Source: CAD feature listing. Evaluate the final solid. Frame: model axes, mm. A direction names the side the tool comes from. Coordinates: 2 decimals unless noted, no trailing zeros. Order: outer loops, then holes, each group sorted by start corner. A loop starts at its lowest first (then second) coordinate and runs counter-clockwise, first axis right, second up.
Item 1: Section B-B on y = 52.5. Return the cut outline in (x, z), then the cut area to 3 significant figures.
Item 2: Ray query, line 1 (X direction, y = 29, z = 128); line 2 (Y direction, x = 14.5, z = 134.5); line 3 (Y direction, x = 21, z = 20). Return the intervals inside material, ascending.
Item 3: Contact query for flat-ended pins moving along their axis: P1, Ø4, axis at x = 22.5, z = 61, coming from the -Y side; P2, Ø1, axis at y = 20.5, z = 53, coming from the -X side; P3, Ø10, axis at y = 1, z = 85.5, coming from the +X side; P4, Ø1.5, axis at x = 21.5, z = 58, coming from the +Y side. Output: stop coordinate, or through.
Item 4: Mould query, pull axis X, two halves, no side actions, for faces 1 (the flat face through (20, 25, 81)), 2 (the flat face through (25, 20, 81)), 3 (the flat face through (22, 50, 81)). Classes: released by +X, released by -X, zero draft, split by the parting line, or undercut.
Item 5: Section A-A on x = 14. Return the cut outline in (y, z).
Item 6: Reachability of faces 4 (the flat face through (20, 55, 79)), 5 (the flat face through (20, -10, 79)), 6 (the flat face through (20, 75, 79)), 7 (the flat face through (22, 30, 79)) from +Z, -Z, +X, -X, +Y, -Y: full face, straight path, thin tool, end or side. Return the list, or none.
Item 7: Section C-C on z = 143. Return the cut outline in (x, y).
Item 8: Section D-D on y = 8. Return the cut outline in (x, z).
from build123d import *

# Parameters (mm, degrees)
BOSS_EXTRUDE1_DEPTH      = 160
SKETCH2_W                = 20
SKETCH2_H                = 160
BOSS_EXTRUDE2_DEPTH      = 30
BOSS_EXTRUDE3_DEPTH      = 10
BOSS_EXTRUDE3_DEPTH_BACK = 10
SKETCH3_W                = 5
SKETCH3_H                = 160
BOSS_EXTRUDE4_DEPTH      = 10
BOSS_EXTRUDE4_DEPTH_BACK = 10
SKETCH4_W                = 5
SKETCH4_H                = 160


with BuildPart() as part:
    # Sketch1 → Boss-Extrude1 (new body)
    with BuildSketch(Plane.XY):
        Polygon((0, 0), (20, 0), (20, 20), (10, 20), (10, 60), (20, 60), (20, 80), (0, 80), align=None)
    extrude(amount=BOSS_EXTRUDE1_DEPTH)

    # Sketch2 → Boss-Extrude2 (add)
    with BuildSketch(Plane.XZ):
        with Locations((10, 80)):
            Rectangle(SKETCH2_W, SKETCH2_H)
    extrude(amount=BOSS_EXTRUDE2_DEPTH)

    # Sketch3 → Boss-Extrude3 (add, two sides: drawn at the far end of the back side and taken through both)
    with BuildSketch(Plane(origin=(0, 20, 0), x_dir=(1, 0, 0), z_dir=(0, 1, 0)).offset(-BOSS_EXTRUDE3_DEPTH_BACK)):
        with Locations((22.5, -80)):
            Rectangle(SKETCH3_W, SKETCH3_H)
    extrude(amount=BOSS_EXTRUDE3_DEPTH + BOSS_EXTRUDE3_DEPTH_BACK)

    # Sketch4 → Boss-Extrude4 (add, two sides: drawn at the far end of the back side and taken through both)
    with BuildSketch(Plane.XZ.offset(-60).offset(-BOSS_EXTRUDE4_DEPTH_BACK)):
        with Locations((22.5, 80)):
            Rectangle(SKETCH4_W, SKETCH4_H)
    extrude(amount=BOSS_EXTRUDE4_DEPTH + BOSS_EXTRUDE4_DEPTH_BACK)


solid = part.part
Answer list:
1. outline: (0, 0) - (10, 0) - (10, 160) - (0, 160) - close; (20, 0) - (25, 0) - (25, 160) - (20, 160) - close
1. area: 2,400 mm2
2. line 1: x = 0 to 10, 20 to 25
2. line 2: y = -30 to 20, 60 to 80
2. line 3: y = 10 to 30, 50 to 70
3. P1: stops at y = 10
3. P2: stops at x = 0
3. P3: stops at x = 20
3. P4: stops at y = 70
4. face 1: undercut
4. face 2: released by +X
4. face 3: zero draft
5. outline: (-30, 0) - (20, 0) - (20, 160) - (-30, 160) - close; (60, 0) - (80, 0) - (80, 160) - (60, 160) - close
6. face 4: +Z, -Z
6. face 5: +Z, -Z, +X, -Y
6. face 6: +Z, -Z, +X, +Y
6. face 7: +Z, -Z, +X
7. outline: (0, -30) - (20, -30) - (20, 10) - (25, 10) - (25, 30) - (20, 30) - (20, 20) - (10, 20) - (10, 60) - (20, 60) - (20, 50) - (25, 50) - (25, 70) - (20, 70) - (20, 80) - (0, 80) - close
8. outline: (0, 0) - (20, 0) - (20, 160) - (0, 160) - close
